```python
from build123d import *

# Parameters (mm, degrees)
SHAPEBINDER_R   = 1.75
PAD020_DEPTH    = 3
SKETCH057_R     = 1.75
PAD021_DEPTH    = 3
POCKET032_DEPTH = 3


with BuildPart() as body:
    # ShapeBinder → Pad020 (new body)
    with BuildSketch(Plane(origin=(-71.291879, -3.78464, 4.5), x_dir=(0, 1, 0), z_dir=(0, 0, 1))):
        with BuildLine():
            Line((44.76589, 42.508121), (44.76589, -71.291879))
            Line((44.76589, -71.291879), (46.11589, -71.291879))
            ThreePointArc((46.11589, -71.291879), (47.86589, -69.541879), (49.61589, -71.291879))
            Line((49.61589, -71.291879), (50.26589, -71.291879))
            Line((50.26589, -71.291879), (50.26589, 47.008121))
            ThreePointArc((50.26589, 47.008121), (49.680103, 48.422335), (48.26589, 49.008121))
            Line((48.26589, 49.008121), (-40.69661, 49.008121))
            ThreePointArc((-40.69661, 49.008121), (-42.110824, 48.422335), (-42.69661, 47.008121))
            Line((-42.69661, 47.008121), (-42.69661, -71.291879))
            Line((-42.69661, -71.291879), (-42.04661, -71.291879))
            ThreePointArc((-42.04661, -71.291879), (-40.29661, -69.541879), (-38.54661, -71.291879))
            Line((-38.54661, -71.291879), (-37.19661, -71.291879))
            Line((-37.19661, -71.291879), (-37.19661, 42.508121))
            ThreePointArc((-37.19661, 42.508121), (-36.903717, 43.215228), (-36.19661, 43.508121))
            Line((-36.19661, 43.508121), (-18.14661, 43.508121))
            ThreePointArc((-18.14661, 43.508121), (-17.439503, 43.215228), (-17.14661, 42.508121))
            Line((-17.14661, 42.508121), (-17.14661, -71.291879))
            Line((-17.14661, -71.291879), (-13.38411, -71.291879))
            Line((-13.38411, -71.291879), (-13.38411, 42.508121))
            ThreePointArc((-13.38411, 42.508121), (-13.091217, 43.215228), (-12.38411, 43.508121))
            Line((-12.38411, 43.508121), (43.76589, 43.508121))
            ThreePointArc((43.76589, 43.508121), (44.472997, 43.215228), (44.76589, 42.508121))
        make_face()
        with Locations((-40.29661, 38.508121)):
            Circle(SHAPEBINDER_R, mode=Mode.SUBTRACT)
        with Locations((47.86589, 38.508121)):
            Circle(SHAPEBINDER_R, mode=Mode.SUBTRACT)
    extrude(amount=PAD020_DEPTH)

    # Sketch057 (on Face26 of Pad020) → Pad021 (join)
    with BuildSketch(Plane.XY.offset(7.5)):
        with Locations((-109.8, -44.08125)):
            Circle(SKETCH057_R)
        with Locations((-109.8, 44.08125)):
            Circle(SKETCH057_R)
        with BuildLine():
            ThreePointArc((0, 45.83125), (-1.75, 44.08125), (0, 42.33125))
            Line((0, 45.83125), (0, 42.33125))
        make_face()
        with BuildLine():
            ThreePointArc((0, -42.33125), (-1.75, -44.08125), (0, -45.83125))
            Line((0, -45.83125), (0, -42.33125))
        make_face()
    extrude(amount=-PAD021_DEPTH)

    # Sketch058 (on Face20 of Pad021) → Pocket032 (cut)
    with BuildSketch(Plane.XY.offset(7.5)):
        with BuildLine():
            ThreePointArc((-118.3, 48.48125), (-121.128427, 47.309677), (-122.3, 44.48125))
            Line((-122.3, -44.48125), (-122.3, 44.48125))
            ThreePointArc((-122.3, -44.48125), (-121.128427, -47.309677), (-118.3, -48.48125))
            Line((2, -48.48125), (-118.3, -48.48125))
            Line((2, 48.48125), (2, -48.48125))
            Line((-118.3, 48.48125), (2, 48.48125))
        make_face()
        with BuildLine():
            ThreePointArc((-118.3, 46.38125), (-119.643503, 45.824753), (-120.2, 44.48125))
            Line((-120.2, 44.48125), (-120.2, -44.48125))
            ThreePointArc((-120.2, -44.48125), (-119.643503, -45.824753), (-118.3, -46.38125))
            Line((-118.3, -46.38125), (0, -46.38125))
            Line((0, -46.38125), (0, 46.38125))
            Line((0, 46.38125), (-118.3, 46.38125))
        make_face(mode=Mode.SUBTRACT)
    extrude(amount=-POCKET032_DEPTH, mode=Mode.SUBTRACT)


with BuildPart() as part_mirroring003:
    # Part__Mirroring003: instance of Body
    add(body.part.mirror(Plane(origin=(0, 0, 0), x_dir=(0, -1, 0), z_dir=(1, 0, 0))))


with BuildPart() as case_inlay:
    # Fusion003 base: copy of Body
    add(body.part)

    # Fusion003: union Part__Mirroring003
    add(part_mirroring003.part)


solid = case_inlay.part
```
CAD build for the part. Positions are in the model's coordinates, mm. Round coordinates to 2 decimals unless told otherwise and drop trailing zeros. Order: outer loops, then holes, each group sorted by start corner. A loop starts at its lowest first (then second) coordinate and runs counter-clockwise, first axis right, second up.
Item 1: Probe line 1 along Y through (x, z) = (-109, 5.05); line 2 along X through (y, z) = (10, 5.45). List the from-to ranges inside material, lowest first.
Item 2: Saw through at A-A on y = 7. Write the cut outline in (x, z).
Item 3: Saw through at C-C on z = 6.3. Write the cut outline in (x, y), then the cut area to 3 significant figures.
Item 4: Saw through at B-B on x = 74.5. Write the cut outline in (y, z).
Reported:
1. line 1: y = -46.38 to -40.98, -20.93 to -17.17, 40.98 to 46.38
1. line 2: x = -120.2 to -114.8, 114.8 to 120.2
2. outline: (-120.2, 4.5) - (-114.8, 4.5) - (-114.8, 7.5) - (-120.2, 7.5) - close; (114.8, 4.5) - (120.2, 4.5) - (120.2, 7.5) - (114.8, 7.5) - close
3. outline: (-120.2, -44.48) arc R1.9 ccw to (-118.3, -46.38) - (118.3, -46.38) arc R1.9 ccw to (120.2, -44.48) - (120.2, 44.48) arc R1.9 ccw to (118.3, 46.38) - (-118.3, 46.38) arc R1.9 ccw to (-120.2, 44.48) - close; hole (-114.8, -39.98) arc R1 ccw to (-113.8, -40.98) - (113.8, -40.98) arc R1 ccw to (114.8, -39.98) - (114.8, -21.93) arc R1 ccw to (113.8, -20.93) - (-113.8, -20.93) arc R1 ccw to (-114.8, -21.93) - close; hole (-114.8, -16.17) arc R1 ccw to (-113.8, -17.17) - (113.8, -17.17) arc R1 ccw to (114.8, -16.17) - (114.8, 39.98) arc R1 ccw to (113.8, 40.98) - (-113.8, 40.98) arc R1 ccw to (-114.8, 39.98) - close
3. area: 4,340 mm2
4. outline: (-46.38, 4.5) - (-40.98, 4.5) - (-40.98, 7.5) - (-46.38, 7.5) - close; (-20.93, 4.5) - (-17.17, 4.5) - (-17.17, 7.5) - (-20.93, 7.5) - close; (40.98, 4.5) - (46.38, 4.5) - (46.38, 7.5) - (40.98, 7.5) - close
